The model under review builds one solid part; all positions refer to its coordinate system, in mm. A direction names the side the tool comes from. Give positions to 0.01 mm unless a question says otherwise; leave off trailing zeros. Order: outer loops, then holes, each group sorted by start corner. A loop starts at its lowest first (then second) coordinate and runs counter-clockwise, first axis right, second up. Notation, with made-up numbers: (71, 21.5) - (97, 21.5) arc R4 cw to (97, 26.5) - close; hole circle Ø6 at (22, -31.5). An arc over 180 degrees is marked (long way). Put each result on its own line as item: value.
Solid Edge part; units mm, degrees
sketch "Sketch1" plane through (0, 0, 0) normal (0, 0, 1) x (1, 0, 0)
  line L0 (-8.5, -15.5) -> (8.5, -15.5)
  line L1 (8.5, -15.5) -> (8.5, 15.5)
  line L2 (8.5, 15.5) -> (-8.5, 15.5)
  line L3 (-8.5, 15.5) -> (-8.5, -15.5)
  dimension "D1" = 8.5
  dimension "D2" = 8.5
extrude "Protrusion1" add sketch "Sketch1" along normal blind 6
sketch "Sketch2" plane through (0, 0, 0) normal (0, 0, -1) x (1, 0, 0)
  line L0 (-1.6, -15.5) -> (1.6, -15.5)
  line L1 (1.6, -15.5) -> (1.6, 15.5)
  line L2 (1.6, 15.5) -> (-1.6, 15.5)
  line L3 (-1.6, 15.5) -> (-1.6, -15.5)
  dimension "D1" = 1.6
extrude "ExtrudedCutout_1" cut sketch "Sketch2" against normal blind 2.4
sketch "Sketch3" plane through (0, 0, 6) normal (0, 0, 1) x (1, 0, 0)
  circle A0 centre (-6, 6.5) radius 1.3
  circle A1 centre (-6, -6.5) radius 1.3
  circle A2 centre (6, -6.5) radius 1.3
  circle A3 centre (6, 6.5) radius 1.3
extrude "Cutout1" cut sketch "Sketch3" against normal up to next
(1) The part is to be moulded in two halves that separate along X. For faces 1 (the cylindrical face through (7.2, -7, 3)), 2 (the flat face through (0, 15.5, 3)), 3 (the flat face through (-8.5, 0, 3)), say which applies: pulls with the +X half, pulls with the -X half, needs draft (parallel to the pull), parting line crosses it, or undercut.
The answers:
face 1: undercut
face 2: needs draft
face 3: pulls with the -X half
(2) Take a section at A-A, the plane z = 0.65. Write out the cut boundary in (x, y).
The answers:
outline: (-8.5, -15.5) - (-1.6, -15.5) - (-1.6, 15.5) - (-8.5, 15.5) - close; (1.6, -15.5) - (8.5, -15.5) - (8.5, 15.5) - (1.6, 15.5) - close; hole circle Ø2.6 at (-6, -6.5); hole circle Ø2.6 at (-6, 6.5); hole circle Ø2.6 at (6, -6.5); hole circle Ø2.6 at (6, 6.5)
(3) Take a section at C-C, the plane y = 7. Write out the cut boundary in (x, z).
The answers:
outline: (-8.5, 0) - (-7.2, 0) - (-7.2, 6) - (-8.5, 6) - close; (-4.8, 0) - (-1.6, 0) - (-1.6, 2.4) - (1.6, 2.4) - (1.6, 0) - (4.8, 0) - (4.8, 6) - (-4.8, 6) - close; (7.2, 0) - (8.5, 0) - (8.5, 6) - (7.2, 6) - close
(4) Take a section at B-B, the plane x = -6. Write out the cut boundary in (y, z).
The answers:
outline: (-15.5, 0) - (-7.8, 0) - (-7.8, 6) - (-15.5, 6) - close; (-5.2, 0) - (5.2, 0) - (5.2, 6) - (-5.2, 6) - close; (7.8, 0) - (15.5, 0) - (15.5, 6) - (7.8, 6) - close
(5) Take a section at D-D, the plane y = -6.5. Write out the cut boundary in (x, z).
The answers:
outline: (-8.5, 0) - (-7.3, 0) - (-7.3, 6) - (-8.5, 6) - close; (-4.7, 0) - (-1.6, 0) - (-1.6, 2.4) - (1.6, 2.4) - (1.6, 0) - (4.7, 0) - (4.7, 6) - (-4.7, 6) - close; (7.3, 0) - (8.5, 0) - (8.5, 6) - (7.3, 6) - close
(6) Wall thickness on L1, parallel to Y at x = 6, z = 2.65; L2, parallel to X at y = -12, z = 1.9; L3, parallel to Y at x = 5.5, z = 2.9: over which ranges is each line inside the solid? List them lowest first.
The answers:
L1: -15.5 to -7.8, -5.2 to 5.2, 7.8 to 15.5
L2: -8.5 to -1.6, 1.6 to 8.5
L3: -15.5 to -7.7, -5.3 to 5.3, 7.7 to 15.5
(7) For faces 4 (the flat face through (0, 0, 6)), 5 (the flat face through (1.6, 0, 1)), list the 3-axis set-ups (+Z, -Z, +X, -X, +Y, -Y) from which the entire face can be reached by the end or side of a thin tool; tool diameter is ignored.
The answers:
face 4: +Z, +X, -X, +Y, -Y
face 5: -Z, +Y, -Y
(8) Clearance check with a flat-ended pin moving along its axis: pin 1 Ø2.5 at (x, y) = (-6, 6.5) entering from +Z. State where the tip first meets the part, or that it passes through.
The answers:
pin 1: through
